Read the model definition and answer for the solid it produces. Units are mm, in the model's axes. A direction names the side the tool comes from. Coordinates: 2 decimals unless noted, no trailing zeros. Order: outer loops, then holes, each group sorted by start corner. A loop starts at its lowest first (then second) coordinate and runs counter-clockwise, first axis right, second up. Notation, with made-up numbers: (-1, 38) - (27, 38) arc R21 ccw to (27, 49) - close; hole circle Ø11 at (40, 42.5). An arc over 180 degrees is marked (long way). Write item = value, one per line.
from build123d import *

# Parameters (mm, degrees)
ESQUISSE1_R        = 7.5
BOSS_EXTRU_1_DEPTH = 12.5
ESQUISSE2_W        = 1.1
ESQUISSE2_H        = 0.35
CHANFREIN1_SIZE    = 1
CHANFREIN1_SIZE2   = 0.5
CHANFREIN2_SIZE    = 0.5
CHANFREIN2_SIZE2   = 1
CHANFREIN3_SIZE    = 0.5


with BuildPart() as part:
    # Esquisse1 → Boss.-Extru.1 (new body, symmetric)
    with BuildSketch(Plane.XY):
        Circle(ESQUISSE1_R)
        with BuildLine():
            Line((3.866903212, 4.574009993), (2.452689649, 3.159796431))
            ThreePointArc((2.452689649, 3.159796431), (1.530733729, 3.69551813), (0.5, 3.968626967))
            Line((0.5, 3.968626967), (0.5, 5.968626967))
            Line((0.5, 5.968626967), (-0.5, 5.968626967))
            Line((-0.5, 5.968626967), (-0.5, 3.968626967))
            ThreePointArc((-0.5, 3.968626967), (-1.530733729, 3.69551813), (-2.452689649, 3.159796431))
            Line((-2.452689649, 3.159796431), (-3.866903212, 4.574009993))
            Line((-3.866903212, 4.574009993), (-4.574009993, 3.866903212))
            Line((-4.574009993, 3.866903212), (-3.159796431, 2.452689649))
            ThreePointArc((-3.159796431, 2.452689649), (-3.69551813, 1.530733729), (-3.968626967, 0.5))
            Line((-3.968626967, 0.5), (-5.968626967, 0.5))
            Line((-5.968626967, 0.5), (-5.968626967, -0.5))
            Line((-5.968626967, -0.5), (-3.968626967, -0.5))
            ThreePointArc((-3.968626967, -0.5), (-3.69551813, -1.530733729), (-3.159796431, -2.452689649))
            Line((-3.159796431, -2.452689649), (-4.574009993, -3.866903212))
            Line((-4.574009993, -3.866903212), (-3.866903212, -4.574009993))
            Line((-3.866903212, -4.574009993), (-2.452689649, -3.159796431))
            ThreePointArc((-2.452689649, -3.159796431), (-1.530733729, -3.69551813), (-0.5, -3.968626967))
            Line((-0.5, -3.968626967), (-0.5, -5.968626967))
            Line((-0.5, -5.968626967), (0.5, -5.968626967))
            Line((0.5, -5.968626967), (0.5, -3.968626967))
            ThreePointArc((0.5, -3.968626967), (1.530733729, -3.69551813), (2.452689649, -3.159796431))
            Line((2.452689649, -3.159796431), (3.866903212, -4.574009993))
            Line((3.866903212, -4.574009993), (4.574009993, -3.866903212))
            Line((4.574009993, -3.866903212), (3.159796431, -2.452689649))
            ThreePointArc((3.159796431, -2.452689649), (3.69551813, -1.530733729), (3.968626967, -0.5))
            Line((3.968626967, -0.5), (5.968626967, -0.5))
            Line((5.968626967, -0.5), (5.968626967, 0.5))
            Line((5.968626967, 0.5), (3.968626967, 0.5))
            ThreePointArc((3.968626967, 0.5), (3.69551813, 1.530733729), (3.159796431, 2.452689649))
            Line((3.159796431, 2.452689649), (4.574009993, 3.866903212))
            Line((4.574009993, 3.866903212), (3.866903212, 4.574009993))
        make_face(mode=Mode.SUBTRACT)
    extrude(amount=BOSS_EXTRU_1_DEPTH, both=True)

    # Esquisse2 → Enlèvement de matière-Révolution1 (revolve, cut)
    with BuildSketch(Plane(origin=(0, 0, 0), x_dir=(0, 0, -1), z_dir=(1, 0, 0))):
        with Locations((-8.2, 7.325)):
            Rectangle(ESQUISSE2_W, ESQUISSE2_H)
        with Locations((8.2, 7.325)):
            Rectangle(ESQUISSE2_W, ESQUISSE2_H)
    revolve(axis=Axis((0, 0, 12.5), (0, 0, -1)), mode=Mode.SUBTRACT)

    # Chanfrein1
    chanfrein1_edges = [part.edges().sort_by_distance(p)[0] for p in [
        (-7.5, 0, 12.5),
    ]]
    chanfrein1_side = [part.faces().sort_by_distance(p)[0] for p in [
        (-7.5, 0, 10.625),
    ]]
    chamfer(chanfrein1_edges, length=CHANFREIN1_SIZE, length2=CHANFREIN1_SIZE2, reference=chanfrein1_side[0])

    # Chanfrein2
    chanfrein2_edges = [part.edges().sort_by_distance(p)[0] for p in [
        (-7.5, 0, -12.5),
    ]]
    chanfrein2_side = [part.faces().sort_by_distance(p)[0] for p in [
        (-7.287867966, 0, -12.5),
    ]]
    chamfer(chanfrein2_edges, length=CHANFREIN2_SIZE, length2=CHANFREIN2_SIZE2, reference=chanfrein2_side[0])

    # Chanfrein3
    chanfrein3_edges = [part.edges().sort_by_distance(p)[0] for p in [
        (-1.530733729, 3.69551813, -12.5),
        (-3.69551813, 1.530733729, -12.5),
        (-3.69551813, -1.530733729, -12.5),
        (-1.530733729, -3.69551813, -12.5),
        (1.530733729, -3.69551813, -12.5),
        (3.69551813, -1.530733729, -12.5),
        (3.69551813, 1.530733729, -12.5),
        (1.530733729, 3.69551813, -12.5),
        (-1.530733729, 3.69551813, 12.5),
        (-3.69551813, 1.530733729, 12.5),
        (-3.69551813, -1.530733729, 12.5),
        (-1.530733729, -3.69551813, 12.5),
        (1.530733729, -3.69551813, 12.5),
        (3.69551813, -1.530733729, 12.5),
        (3.69551813, 1.530733729, 12.5),
        (1.530733729, 3.69551813, 12.5),
    ]]
    chamfer(chanfrein3_edges, length=CHANFREIN3_SIZE)


solid = part.part
1) For faces 1 (the face through (-1.52, 3.7, 0.17)), 2 (the face through (-1.64, -3.92, 12.25)), 3 (the face through (7.09, -0.93, -8.21)), determine the directions among +Z, -Z, +X, -X, +Y, -Y from which every point of the face is accessible in a straight line to the end or side of a thin tool.
Returned:
face_1 = +Z, -Z
face_2 = +Z
face_3 = none
2) Straight lines are drawn through the part: line 1 along Z through (x, y) = (6.75, 3); line 2 along X through (y, z) = (-4.25, -2); line 3 along Y through (x, z) = (-0.25, 4.5). For each, find the intervals that lie inside material, in ascending order. Write a range as from..to.
Returned:
line_1 = -11.73..-8.75, -7.65..7.65, 8.75..11.73
line_2 = -6.18..-4.19, -3.54..-0.5, 0.5..3.54, 4.19..6.18
line_3 = -7.5..-5.97, 5.97..7.5
3) The part is cut by section A-A (y = 0). Determine the outline of the cut face in (x, z).
Returned:
outline = (-7.5, -11.5) - (-7, -12.5) - (-5.97, -12.5) - (-5.97, 12.5) - (-7, 12.5) - (-7.5, 11.5) - (-7.5, 8.75) - (-7.15, 8.75) - (-7.15, 7.65) - (-7.5, 7.65) - (-7.5, -7.65) - (-7.15, -7.65) - (-7.15, -8.75) - (-7.5, -8.75) - close; (5.97, -12.5) - (7, -12.5) - (7.5, -11.5) - (7.5, -8.75) - (7.15, -8.75) - (7.15, -7.65) - (7.5, -7.65) - (7.5, 7.65) - (7.15, 7.65) - (7.15, 8.75) - (7.5, 8.75) - (7.5, 11.5) - (7, 12.5) - (5.97, 12.5) - close
4) Determine the mould class of faces 4 (the face through (1, -5, 12.5)), 5 (the face through (-3.877, 3.17, 0.175)), 6 (the face through (7.154, 2.253, 0.107)) for opening direction X: pulls with the +X half, pulls with the -X half, needs draft (parallel to the pull), parting line crosses it, or undercut.
Returned:
face_4 = needs draft
face_5 = undercut
face_6 = parting line crosses it
5) Flat-ended cylindrical pins translate along their axes: pin 1 Ø2 at (x, z) = (-5.5, 2) entering from +Y; pin 2 Ø1.6 at (y, z) = (-5.5, 4.5) entering from +X; pin 3 Ø1.6 at (y, z) = (-5, 5.5) entering from -X; pin 4 Ø4.5 at (x, y) = (0, 0) entering from +Z. Find the tip coordinate at first contact, or state that the pin passes through.
Returned:
pin_1 = 6
pin_2 = 5.84
pin_3 = -6.21
pin_4 = through
